Autodesk Inventor part; units mm, degrees
ref_plane "YZ Plane" through (0, 0, 0) normal (1, 0, 0) x (0, 1, 0)
ref_plane "XZ Plane" through (0, 0, 0) normal (0, 1, 0) x (-1, 0, 0)
ref_plane "XY Plane" through (0, 0, 0) normal (0, 0, 1) x (1, 0, 0)
ref_plane "Płaszczyzna konstrukcyjna1" through (-2.3844, -12.525, -22.8032) normal (1, 0, 0) x (0, 1, 0)
sketch "Szkic1" plane through (-2.3844, -12.525, -22.8032) normal (1, 0, 0) x (0, 1, 0)
  circle A0 centre (0, 0) radius 3
  point P0 (12.525, 22.8032)
  dimension "d0" = 6
extrude "Wyciągnięcie proste1" add sketch "Szkic1" along normal blind 60
sketch "Szkic2" plane through (-2.3844, -12.525, -22.8032) normal (-1, 0, 0) x (0, 0, 1)
  line L0 (33, -7.4436) -> (-7, -7.4436)
  line L1 (-7, -7.4436) -> (-7, 7.5564)
  line L2 (-7, 7.5564) -> (33, 7.5564)
  line L3 (33, 7.5564) -> (33, -7.4436)
  line L4 (33, -7.4436) -> (-7, 7.5564) construction
  line L5 (-7, -7.4436) -> (33, 7.5564) construction
  line L6 (0, 16.5188) -> (0, -11.4374)
  circle A0 centre (0, 0) radius 3
  point P0 (22.8032, 12.525)
  point P1 (13, 0.0564)
  dimension "d3" = 40
  dimension "d4" = 15
  dimension "d5" = 7
extrude "Wyciągnięcie proste2" add sketch "Szkic2" along normal blind 1.5
full round fillet "Zaokrąglenie1" first side at (-2.8844, -19.9687, -16.4698) centre faces at (-2.8844, -9.9687, -29.8032) second side at (-2.8844, -4.9687, -3.1365)
full round fillet "Zaokrąglenie2" first side at (-2.8844, -19.9687, -11.4699) centre faces at (-2.8844, -14.9687, 10.1968) second side at (-2.8844, -4.9687, -0.6365)
properties part number "uchwyt1" material "Aluminium 3004-O"
For this review, take the finished solid that the model builds, in its own axes (mm). Coordinates: 2 decimals unless noted, no trailing zeros. Loops run counter-clockwise (first coordinate to the right, second up) from the corner with the lowest first, then second, coordinate; pieces in that order, holes last. Notation, with made-up numbers: (38.25, 80.5) - (92.25, 80.5) arc R19 ccw to (92.25, 101.5) - close; hole circle Ø3 at (47.5, 89.5). An arc over 180 degrees is marked (long way). Use a Markdown table: item, result. Add a question column.
Item 1: We need section D-D (z = -16). Give the boundary of the cut face in (x, y), and give its area (3 significant figures).
Item 2: For line 1 (X direction, y = -17.75, z = -25); line 2 (Y direction, x = 15, z = -23); line 3 (Z direction, x = 6, y = -12.75), list the stretches that pass through material, from the lowest coordinate up.
Item 3: Insertion check: pin 1 Ø4.5 at (y, z) = (-9.5, -16.5) entering from +X; pin 2 Ø3 at (x, z) = (39, -20) entering from +Y; pin 3 Ø2 at (x, y) = (23.5, -11) entering from +Z. Each pin has a flat end and moves straight along its axis. Give the tip position at first contact, or say it passes through.
Item 4: We need section C-C (x = 33.5). Give the boundary of the cut face in (y, z) (3 decimals), and give its area (3 significant figures).
Item 5: We need section A-A (z = -24). Give the boundary of the cut face in (x, y), and give its area (3 significant figures).
Item 6: We need section B-B (y = -17.25). Give the boundary of the cut face in (x, z).
Item 7: Mouldability with a two-part tool opening along X and no side actions: class faces 1 (the face through (27.2, -15.52, -22.94)), 2 (the face through (-3.884, -12, -10)), 3 (the face through (57.616, -13, -23)) as pulls with the +X half, pulls with the -X half, needs draft (parallel to the pull), parting line crosses it, or undercut.
Results list:
| question | item | result |
|---|---|---|
| 1 | outline | (-3.88, -19.97) - (-2.38, -19.97) - (-2.38, -4.97) - (-3.88, -4.97) - close |
| 1 | area | 22.5 mm^2 |
| 2 | line 1 | x = -3.88 to -2.38 |
| 2 | line 2 | y = -15.52 to -9.53 |
| 2 | line 3 | z = -25.79 to -19.81 |
| 3 | pin 1 | stops at x = -2.38 |
| 3 | pin 2 | stops at y = -9.82 |
| 3 | pin 3 | stops at z = -19.85 |
| 4 | outline | circle Ø6 at (-12.525, -22.803) |
| 4 | area | 28.3 mm^2 |
| 5 | outline | (-3.88, -19.77) - (-2.38, -19.77) - (-2.38, -15.28) - (57.62, -15.28) - (57.62, -9.77) - (-2.38, -9.77) - (-2.38, -5.16) - (-3.88, -5.16) - close |
| 5 | area | 352 mm^2 |
| 6 | outline | (-3.88, -28.08) - (-2.38, -28.08) - (-2.38, 8.48) - (-3.88, 8.48) - close |
| 7 | face 1 | needs draft |
| 7 | face 2 | pulls with the -X half |
| 7 | face 3 | pulls with the +X half |
